Autodesk Inventor part; units mm, degrees
ref_plane "YZ Plane" through (0, 0, 0) normal (1, 0, 0) x (0, 1, 0)
ref_plane "XZ Plane" through (0, 0, 0) normal (0, 1, 0) x (-1, 0, 0)
ref_plane "XY Plane" through (0, 0, 0) normal (0, 0, 1) x (1, 0, 0)
sketch "Sketch4" plane through (0, 0, 0) normal (0, 0, 1) x (1, 0, 0)
  line L0 (-3.7, 0) -> (16, 0)
  line L1 (0, 0) -> (-3.7, 0)
  line L2 (0, 4.75) -> (0, 3.25)
  line L3 (0.8, 2.45) -> (0.8, 2.45)
  line L4 (0.8, 2.45) -> (1.6, 2.5)
  arc A0 (0, 3.25) -> (0.8, 2.45) centre (0.8, 3.25) ccw
  line L5 (-3.7, 0) -> (-3.7, 2.5)
  line L6 (0, 4.75) -> (-2.0492, 4.75)
  arc A1 (-2.0492, 4.75) -> (-3.7, 2.5) centre (3.4767, -1.0349) ccw
  line L7 (1.6, 2.5) -> (16, 2.5)
  line L8 (16, 2.5) -> (16, 0)
  point P0 (0, 2.45)
  dimension "d71" = 0.8
  dimension "d72" = 16
  dimension "d74" = 0.8
  dimension "d75" = 4.9
  dimension "d78" = 5
  dimension "d82" = 8
  dimension "d83" = 3.7
  dimension "d84" = 9.5
  dimension "d104" = 14.4
  dimension "d105" = 5
revolve "Revolution7" add sketch "Sketch4" angle 360 about axis through (-3.7, 0, 0) along (1, 0, 0)
sketch "Sketch5" plane through (-3.7, 0, 0) normal (-1, 0, 0) x (0, 0, 1)
  circle A0 centre (0, 0) radius 2.25 construction
  circle A1 centre (0, 0) radius 1.575 construction
  line L0 (0, 0) -> (-1.364, 0.7875)
  line L1 (0, 0) -> (-1.364, -0.7875)
  line L2 (-1.8008, 0) -> (1.7887, 0)
  line L3 (-2.25, 0) -> (-1.364, -0.7875)
  line L4 (-2.25, 0) -> (-1.364, 0.7875)
  dimension "d88" = 4.5
  dimension "d89" = 3.15
  dimension "d90" = 30
  dimension "d91" = 30
extrude "Extrusion1" cut sketch "Sketch5" against normal blind 1.91
pattern_circular "Circular Pattern1" count 6 over 360 about axis through (-10, 0, 0) along (1, 0, 0) of "Extrusion1"
fillet "Fillet1" radius 0.45 12 edges at (-2.745, -1.9486, -1.125) (-2.745, -0.7875, -1.364) (-2.745, -1.575, 0) (-2.745, -1.9486, 1.125) (-2.745, -0.7875, 1.364) (-2.745, 0, 2.25) (-2.745, 1.575, 0) (-2.745, 1.9486, 1.125) (-2.745, 0.7875, 1.364) (-2.745, 0.7875, -1.364) (-2.745, 0, -2.25) (-2.745, 1.9486, -1.125)
thread "Thread7"
properties part number "Винты со звездообразным углублением в плоско-выпуклой головке ISO 14583 — M5 x 16 — 4.8" material "Сталь"
Check sheet for the modelled part. Datum: model origin and axes. Units: mm. A direction names the side the tool comes from. Give positions to 0.01 mm unless a question says otherwise; leave off trailing zeros. Order: outer loops, then holes, each group sorted by start corner. A loop starts at its lowest first (then second) coordinate and runs counter-clockwise, first axis right, second up. Notation, with made-up numbers: (32, 58) -> (79, 58) arc R16 cw to (79, 79) -> close; hole circle Ø1 at (28, 8.25). An arc over 180 degrees is marked (long way). Return JSON: item names as keys, results as strings.
1. Set-up check for faces 4 (the flat face through (0, 2, -3)), 5 (the cylindrical face through (-1.039, 2.192, 4.214)): record each of +Z, -Z, +X, -X, +Y, -Y from which the full face is reachable in a straight line by a thin tool's end or side.
From the geometry:
{"face 4": "+X", "face 5": "+X, -X"}
2. Material ranges on probe 1 along X at (y, z) = (-1.25, -0.5); probe 2 along X at (y, z) = (-3, -2.75); probe 3 along Y at (x, z) = (5.25, -0.25), recorded low to high. Write a range as [from, to].
From the geometry:
{"probe 1": "[-1.79, 16]", "probe 2": "[-2.68, 0]", "probe 3": "[-2.49, 2.49]"}
3. Cross-section at A-A, the plane x = 6. Record the cut outline in (y, z).
From the geometry:
{"outline": "circle Ø5 at (0, 0)"}
4. Mould release check, pull along Y, two halves, no side actions. Record for faces 1 (the flat face through (-3.7, 2, 0)), 2 (the flat face through (-1.79, 0, 0)), 3 (the conical face through (1.028, -1.956, -1.499)): +Y half, -Y half, draft (parallel to the pull), parting line (faces both ways), or undercut.
From the geometry:
{"face 1": "draft", "face 2": "undercut", "face 3": "parting line"}
5. Go/stop test with flat-tipped pins: P1, Ø1, axis at x = 8.5, z = 3.5, coming from the +Y side; P2, Ø1.5, axis at y = -3.5, z = 0.5, coming from the +X side; P3, Ø5, axis at x = 12.5, z = 2, coming from the +Y side; P4, Ø2, axis at x = 3, z = 1.5, coming from the +Y side. Record where each tip stops, or that it passes through.
From the geometry:
{"P1": "through", "P2": "x = 0.15", "P3": "y = 2.5", "P4": "y = 2.45"}
6. Cross-section at B-B, the plane x = -0.25. Record the cut outline in (y, z), plus the area to 3 significant figures.
From the geometry:
{"outline": "circle Ø9.5 at (0, 0)", "area": "70.9 mm^2"}
